The model under review builds one solid part; all positions refer to its coordinate system, in mm. A direction names the side the tool comes from. Give positions to 0.01 mm unless a question says otherwise; leave off trailing zeros. Order: outer loops, then holes, each group sorted by start corner. A loop starts at its lowest first (then second) coordinate and runs counter-clockwise, first axis right, second up. Notation, with made-up numbers: (11.5, -18.5) - (52.5, -18.5) arc R28 ccw to (52.5, 4.5) - close; hole circle Ø5 at (1.25, -32.5). An arc over 180 degrees is marked (long way). Use CSV: the item, a comma, the result in double quotes. Start each with the question number.
1. Take a section at B-B, the plane y = -7.5. State the section outline as (x, z) points.
2. Take a section at C-C, the plane x = 4.5. State the section outline as (y, z) points, then the cut area to 3 significant figures.
3. Machinability: for faces 4 (the flat face through (-4.232, -9.1, 13.2)), 5 (the flat face through (-6.032, -7, 15)), which of the approach directions +Z, -Z, +X, -X, +Y, -Y give a long, thin tool a straight path to every point of the face, cutting with its end or side? Answer none if there is none.
4. Take a section at D-D, the plane y = -3.25. State the section outline as (x, z) points, then the cut area to 3 significant figures.
5. Take a section at A-A, the plane z = 11. State the section outline as (x, y) points, then the cut area to 3 significant figures.
6. For pin 1 (3 mm diameter, centred on y = -7.5, z = 11, fed in from -X); pin 2 (7.5 mm diameter, centred on x = 8.5, y = -4, fed in from +Z), all flat-tipped, find the tip position at first contact; note any pin that passes through.
7. To check wall thickness, follow line 1 (Z direction, x = -5.55, y = -7.5); line 2 (Z direction, x = 2.75, y = -11.75); line 3 (X direction, y = -12.25, z = 15.25). State the ranges of each line that lie inside material, in increasing order. Write a range as [from, to].
8. Draft analysis for pull direction Y (two halves, no side actions). For faces 1 (the cylindrical face through (-5.12, -7.83, 21.48)), 2 (the flat face through (-5, -7, 25)), 3 (the flat face through (-5, 0, 7)), state which applies: released by +Y, released by -Y, zero draft, split by the parting line, or undercut.
```python
from build123d import *

# Parameters (mm, degrees)
F0_W           = 1.8
F0_H           = 1.7999967287
F0_W_2         = 23.2
F0_H_2         = 23.2000032713
F1_DEPTH       = 15
F4_D           = 5
F4_DEPTH       = 1.8
F4_TIP         = 1.5021515476
F4_ON_F3_D     = 5
F4_ON_F3_DEPTH = 1.8
F4_ON_F3_TIP   = 1.5021515476


with BuildPart() as f1:
    # F0 (on Front) → F1 (new body)
    with BuildSketch(Plane.XZ):
        with Locations((-5.1324295796, 0.8999983644)):
            Rectangle(F0_W, F0_H)
        with Locations((7.3675704204, 0.8999983644)):
            Rectangle(F0_W_2, F0_H)
        with Locations((-5.1324295796, 13.3999983644)):
            Rectangle(F0_W, F0_H_2)
    extrude(amount=F1_DEPTH)

    # F4
    with Locations(Plane(origin=(-6.0324295796, 0, 0), x_dir=(0, -1, 0), z_dir=(-1, 0, 0))):
        with Locations((7.5, 19), (7.5, 11)):
            Hole(F4_D / 2, depth=F4_DEPTH)
            with Locations((0, 0, -(F4_DEPTH + F4_TIP / 2))):  # 118° drill point
                Cone(0, F4_D / 2, F4_TIP, mode=Mode.SUBTRACT)

    # F4 on F3
    with Locations(Plane(origin=(0, 0, 0), x_dir=(1, 0, 0), z_dir=(0, 0, -1))):
        with Locations((4.9675704204, 7.5), (12.9675704204, 7.5)):
            Hole(F4_ON_F3_D / 2, depth=F4_ON_F3_DEPTH)
            with Locations((0, 0, -(F4_ON_F3_DEPTH + F4_ON_F3_TIP / 2))):  # 118° drill point
                Cone(0, F4_ON_F3_D / 2, F4_ON_F3_TIP, mode=Mode.SUBTRACT)


solid = f1.part
```
Determined:
1,outline,"(-6.03, 0) - (2.47, 0) - (2.47, 1.8) - (-4.23, 1.8) - (-4.23, 8.5) - (-6.03, 8.5) - close; (-6.03, 13.5) - (-4.23, 13.5) - (-4.23, 16.5) - (-6.03, 16.5) - close; (-6.03, 21.5) - (-4.23, 21.5) - (-4.23, 25) - (-6.03, 25) - close; (7.47, 0) - (10.47, 0) - (10.47, 1.8) - (7.47, 1.8) - close; (15.47, 0) - (18.97, 0) - (18.97, 1.8) - (15.47, 1.8) - close"
2,outline,"(-15, 0) - (-9.96, 0) - (-9.96, 1.8) - (-15, 1.8) - close; (-5.04, 0) - (0, 0) - (0, 1.8) - (-5.04, 1.8) - close"
2,area,"18.2 mm²"
3,face 4,"+Z, +X, +Y, -Y"
3,face 5,"+Z, -Z, -X, +Y, -Y"
4,outline,"(-6.03, 0) - (18.97, 0) - (18.97, 1.8) - (-4.23, 1.8) - (-4.23, 25) - (-6.03, 25) - close"
4,area,"86.8 mm²"
5,outline,"(-6.03, -15) - (-4.23, -15) - (-4.23, -10) - (-6.03, -10) - close; (-6.03, -5) - (-4.23, -5) - (-4.23, 0) - (-6.03, 0) - close"
5,area,"18.0 mm²"
6,pin 1,"passes through"
6,pin 2,"stops at z = 1.8"
7,line 1,"z = [0, 8.5], [13.5, 16.5], [21.5, 25]"
7,line 2,"z = [0, 1.8]"
7,line 3,"x = [-6.03, -4.23]"
8,face 1,"undercut"
8,face 2,"zero draft"
8,face 3,"released by +Y"
